Geometry check sheet. Reference: the model listing, model coordinates, mm. A direction names the side the tool comes from. Coordinates: 2 decimals unless noted, no trailing zeros. Write each loop counter-clockwise with the first axis right and the second up, starting at its lowest first coordinate (ties: lowest second). Pieces come first, ordered by that corner, then holes. Notation, with made-up numbers: (48, 2) -> (102, 2) arc R11 cw to (102, 16) -> close; hole circle Ø1 at (1, 22). An arc over 180 degrees is marked (long way). Put each result on its own line as item: value. Start each with the question number.
from build123d import *

# Parameters (mm, degrees)
BOSS_EXTRUDE1_DEPTH      = 10.1
BOSS_EXTRUDE1_DEPTH_BACK = 10.1
BOSS_EXTRUDE2_DEPTH      = 10


with BuildPart() as part:
    # Sketch1 → Boss-Extrude1 (new, two sides: drawn at the far end of the back side and taken through both)
    with BuildSketch(Plane.XY.offset(-BOSS_EXTRUDE1_DEPTH_BACK)):
        Polygon((0, 0), (0, 150), (25, 150), (25, 109.9), (44.8, 90.1), (5, 90.1), (5, 69.9), (65, 69.9), (65, 49.7), (85.2, 49.7), (56.505691621, 0), align=None)
        Polygon((10, 64.9), (10, 10), (50.732188929, 10), (67.879491924, 39.7), (55, 39.7), (55, 64.9), align=None, mode=Mode.SUBTRACT)
    extrude(amount=BOSS_EXTRUDE1_DEPTH + BOSS_EXTRUDE1_DEPTH_BACK)

    # Sketch2 → Boss-Extrude2 (add)
    with BuildSketch(Plane.XY.offset(10.1)):
        Polygon((44.8, 90.1), (70.8, 90.1), (85.2, 75.7), (85.2, 49.7), (56.505691621, 0), (0, 0), (0, 150), (25, 150), (25, 109.9), align=None)
    extrude(amount=BOSS_EXTRUDE2_DEPTH)


solid = part.part
Item 1: Go/stop test with flat-tipped pins: P1, Ø16, axis at y = 26.5, z = 0, coming from the +X side; P2, Ø1, axis at y = 60.5, z = 7.5, coming from the +X side; P3, Ø4, axis at x = 63, z = 3, coming from the -Y side. Record where each tip stops, or that it passes through.
Item 2: Section check B-B, the plane x = 39.5. Enter the section's corners in (y, z).
Item 3: Section check D-D, the plane y = 83.5. Enter the section's corners in (x, z), and give its area (3 significant figures).
Item 4: Scan lines: line 1 along Y through (x, z) = (22, 4.5); line 2 along X through (y, z) = (51, 6); line 3 along Y through (x, z) = (48, -5). Record each from-to range of solid material in increasing order. Write a range as [from, to].
Item 5: Mould release check, pull along Y, two halves, no side actions. Record for faces 1 (the flat face through (12, 150, 5)), 2 (the flat face through (10, 38, 0)), 3 (the flat face through (34, 59, 20.1)): released by +Y, released by -Y, zero draft, split by the parting line, or undercut.
Item 6: Section check C-C, the plane z = 16. Enter the section's corners in (x, y), and give its area (3 significant figures).
Item 7: Section check A-A, the plane z = 7.5. Enter the section's corners in (x, y).
Item 8: Access from +Z, -Z, +X, -X, +Y, -Y to the whole of each face (thin tool, end or side, straight path). Record for faces 4 (the flat face through (65, 60, 0)), 5 (the flat face through (25, 130, 5)), 6 (the flat face through (55, 52, 0)), 7 (the flat face through (29, 0, 5)), 8 (the flat face through (25, 90.1, 0)).
From the geometry:
1. P1: x = 76.42
1. P2: x = 65
1. P3: y = 7.78
2. outline: (0, -10.1) -> (10, -10.1) -> (10, 10.1) -> (64.9, 10.1) -> (64.9, -10.1) -> (69.9, -10.1) -> (69.9, 10.1) -> (90.1, 10.1) -> (90.1, -10.1) -> (95.4, -10.1) -> (95.4, 20.1) -> (0, 20.1) -> close
3. outline: (0, -10.1) -> (5, -10.1) -> (5, 10.1) -> (77.4, 10.1) -> (77.4, 20.1) -> (0, 20.1) -> close
3. area: 875 mm²
4. line 1: [0, 10], [64.9, 69.9], [90.1, 150]
4. line 2: [0, 10], [55, 65]
4. line 3: [0, 10], [64.9, 69.9]
5. face 1: released by +Y
5. face 2: undercut
5. face 3: zero draft
6. outline: (0, 0) -> (56.51, 0) -> (85.2, 49.7) -> (85.2, 75.7) -> (70.8, 90.1) -> (44.8, 90.1) -> (25, 109.9) -> (25, 150) -> (0, 150) -> close
6. area: 8,550 mm²
7. outline: (0, 0) -> (56.51, 0) -> (85.2, 49.7) -> (65, 49.7) -> (65, 69.9) -> (5, 69.9) -> (5, 90.1) -> (44.8, 90.1) -> (25, 109.9) -> (25, 150) -> (0, 150) -> close; hole (10, 10) -> (50.73, 10) -> (67.88, 39.7) -> (55, 39.7) -> (55, 64.9) -> (10, 64.9) -> close
8. face 4: -Z, +X, +Y
8. face 5: +Z, -Z, +X, +Y
8. face 6: -Z
8. face 7: +Z, -Z, +X, -X, -Y
8. face 8: -Z, +X
